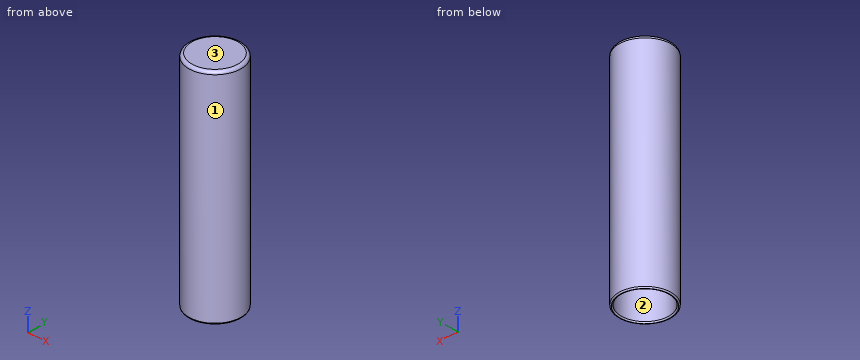
from build123d import *

# Parameters (mm, degrees)
F2_R = 2.54
F3_R = 1.01599


# Not quite as in the source:
# - a fillet or chamfer is up to 0.001 mm smaller than in the source, because OpenCascade refuses the exact size


with BuildPart() as f1:
    # F0 (on Front) → F1 (revolve)
    with BuildSketch(Plane.XZ):
        with BuildLine():
            Line((0, -21.7963978648), (0, 0))
            Line((0, 0), (-22.6568, 0))
            Line((-22.6568, 0), (-22.6568, -190.5))
            Line((-22.6568, -190.5), (-20.6248, -190.5))
            Line((-20.6248, -190.5), (-20.6248, -27.3231199056))
            ThreePointArc((-20.6248, -27.3231199056), (-20.108359218, -25.7879299854), (-18.7690455975, -24.877019343))
            add(Edge.make_bspline(
                [(-18.7690455975, -24.877019343), (-15.7267844832, -24.0260102693), (-9.2902414756, -22.325160199), (-3.2160062892, -21.9794397154), (0, -21.7963978648)],
                knots=[0.0872743239, 0.0872743239, 0.0872743239, 0.0872743239, 0.5167570197, 1, 1, 1, 1], degree=3))
        make_face()
    revolve(axis=Axis((0, 0, -10.8981989324), (0, 0, 1)))

    # F2
    f2_edges = [f1.edges().sort_by_distance(p)[0] for p in [
        (22.6568, 0, 0),
    ]]
    fillet(f2_edges, radius=F2_R)

    # F3 (radius 1.016 in the source; OpenCascade refuses exactly that, so slightly less here)
    f3_edges = [f1.edges().sort_by_distance(p)[0] for p in [
        (22.6568, 0, -190.5),
        (20.6248, 0, -190.5),
    ]]
    fillet(f3_edges, radius=F3_R)


solid = f1.part
Source: CAD feature listing. Evaluate the final solid. Frame: model axes, mm. Face numbers are marked on the shaded views. Give positions to 0.01 mm unless a question says otherwise; leave off trailing zeros. Write each loop counter-clockwise with the first axis right and the second up, starting at its lowest first coordinate (ties: lowest second). Pieces come first, ordered by that corner, then holes. Notation, with made-up numbers: M 3,14 L 43,14 A18 cw 43,38 Z; hole C 31,3 d10. An arc over 180 degrees is marked long. Answer as a JSON object with one key per item and string values.
Q1. Contact query for flat-ended pins moving along their axis: P1, Ø1, axis at x = 13, z = -157.5, coming from the -Y side; P2, Ø8, axis at x = 2.5, y = 8.5, coming from the -Z side; P3, Ø6, axis at y = 16, z = -162, coming from the +X side. Output: stop coordinate, or through.
Geometry check:
{"P1": "stops at y = -18.9", "P2": "stops at z = -23.35", "P3": "stops at x = 18.56"}
Q2. Ray query, line 1 along X through (y, z) = (0, -120); line 2 along Y through (x, z) = (1, -29). Return the intervals inside material, ascending.
Geometry check:
{"line 1": "x = -22.66 to -20.62, 20.62 to 22.66", "line 2": "y = -22.63 to -20.6, 20.6 to 22.63"}
Q3. Cut plane A-A, the plane z = -42.5. Return the cut outline in (x, y).
Geometry check:
{"outline": "C 0,0 d45.31; hole C 0,0 d41.25"}
Q4. Mould query, pull axis X, two halves, no side actions, for the marked faces 1, 2 and 3. Classes: +X half, -X half, draft (parallel to the pull), parting line (faces both ways), or undercut.
Geometry check:
{"face 1": "parting line", "face 2": "undercut", "face 3": "draft"}
